Read the model definition and answer for the solid it produces. Units are mm, in the model's axes. A direction names the side the tool comes from. Coordinates: 2 decimals unless noted, no trailing zeros. Order: outer loops, then holes, each group sorted by start corner. A loop starts at its lowest first (then second) coordinate and runs counter-clockwise, first axis right, second up.
```python
from build123d import *

# Parameters (mm, degrees)
SKETCH_1_W        = 120
SKETCH_1_H        = 80
SKETCH_1_W_2      = 28
SKETCH_1_H_2      = 45
BASE_PLATE_DEPTH  = 4
TABS2_START       = -5
TABS2_DEPTH       = 10
TABS2_2_OUTLINE_W = 26
TABS2_2_OUTLINE_H = 4
TABS2_2_DEPTH     = 1.41096
TABS2_START_2     = 5
TABS2_3_OUTLINE_W = 26
TABS2_3_OUTLINE_H = 4
TABS2_3_DEPTH     = 20
TABS2_START_3     = -13
TABS2_4_DEPTH     = 26
TABS2_5_DEPTH     = 26
HOLES_DEPTH       = 77.321687612
HOLES_DEPTH_BACK  = 77.321687612
SKETCH_10_R       = 4.05
SKETCH_12_W       = 8.2
SKETCH_12_H       = 8.2
HOLE2_DEPTH       = 4
FILLET_2_R        = 10
SKETCH_11_R       = 5.1
MOUNT_HOLES_DEPTH = 4


with BuildPart() as part:
    # Base Plate: sheet metal written as solids
    # Sketch 1 → Base Plate (new body)
    with BuildSketch(Plane.XY):
        Rectangle(SKETCH_1_W, SKETCH_1_H)
        Rectangle(SKETCH_1_W_2, SKETCH_1_H_2, mode=Mode.SUBTRACT)
    extrude(amount=-BASE_PLATE_DEPTH)

    # Tabs2: read off the stored shape, not the designer's step
    # Tabs2 outline → Tabs2 (cut)
    with BuildSketch(Plane.XY.offset(TABS2_START)):
        with BuildLine():
            ThreePointArc((-13, 31.6), (-13.5, 32.1), (-14, 31.6))
            Line((-14, 31.6), (-14, 22.5))
            Line((-14, 22.5), (-13, 22.5))
            Line((-13, 22.5), (-13, 31.6))
        make_face()
        with BuildLine():
            Line((-13, -22.5), (-14, -22.5))
            Line((-14, -22.5), (-14, -31.6))
            ThreePointArc((-14, -31.6), (-13.5, -32.1), (-13, -31.6))
            Line((-13, -31.6), (-13, -22.5))
        make_face()
        with BuildLine():
            Line((13, 31.6), (13, 22.5))
            Line((13, 22.5), (14, 22.5))
            Line((14, 22.5), (14, 31.6))
            ThreePointArc((14, 31.6), (13.5, 32.1), (13, 31.6))
        make_face()
        with BuildLine():
            Line((14, -22.5), (13, -22.5))
            Line((13, -22.5), (13, -31.6))
            ThreePointArc((13, -31.6), (13.5, -32.1), (14, -31.6))
            Line((14, -31.6), (14, -22.5))
        make_face()
    extrude(amount=TABS2_DEPTH, mode=Mode.SUBTRACT)

    # Tabs2 2 outline → Tabs2 2 (cut)
    with BuildSketch(Plane.XY.offset(TABS2_START)):
        with Locations((0, 24.5)):
            Rectangle(TABS2_2_OUTLINE_W, TABS2_2_OUTLINE_H)
        with Locations((0, -24.5)):
            Rectangle(TABS2_2_OUTLINE_W, TABS2_2_OUTLINE_H)
    extrude(amount=TABS2_2_DEPTH, mode=Mode.SUBTRACT)

    # Tabs2 4 outline → Tabs2 4 (cut)
    with BuildSketch(Plane.YZ.offset(TABS2_START_3)):
        with BuildLine():
            ThreePointArc((31.5, -4), (27.257359313, -2.937253933), (24.016685226, 0))
            Line((24.016685226, 0), (22.5, 0))
            Line((22.5, 0), (22.5, -3.58904))
            Line((22.5, -3.58904), (26.5, -3.58904))
            Line((26.5, -3.58904), (26.5, -4))
            Line((26.5, -4), (31.5, -4))
        make_face()
        with BuildLine():
            Line((-22.5, -3.58904), (-22.5, 0))
            Line((-22.5, 0), (-24.016685226, 0))
            ThreePointArc((-24.016685226, 0), (-27.257359313, -2.937253933), (-31.5, -4))
            Line((-31.5, -4), (-26.5, -4))
            Line((-26.5, -4), (-26.5, -3.58904))
            Line((-26.5, -3.58904), (-22.5, -3.58904))
        make_face()
    extrude(amount=TABS2_4_DEPTH, mode=Mode.SUBTRACT)



with BuildPart() as body_2:
    # Tabs2 3 outline → Tabs2 3 (new body)
    with BuildSketch(Plane.XY.offset(TABS2_START_2)):
        with Locations((0, 24.5)):
            Rectangle(TABS2_3_OUTLINE_W, TABS2_3_OUTLINE_H)
        with Locations((0, -24.5)):
            Rectangle(TABS2_3_OUTLINE_W, TABS2_3_OUTLINE_H)
    extrude(amount=TABS2_3_DEPTH)


with BuildPart() as part_1:
    add(part.part)

    add(body_2.part)  # Tabs2 5 merges body 2
    # Tabs2 5 outline → Tabs2 5 (add)
    with BuildSketch(Plane.YZ.offset(TABS2_START_3)):
        with BuildLine():
            Line((26.5, 5), (22.5, 5))
            ThreePointArc((22.5, 5), (22.88751392, 2.38751392), (24.016685226, 0))
            Line((24.016685226, 0), (31.5, 0))
            ThreePointArc((31.5, 0), (27.964466094, 1.464466094), (26.5, 5))
        make_face()
        with BuildLine():
            Line((-31.5, 0), (-24.016685226, 0))
            ThreePointArc((-24.016685226, 0), (-22.88751392, 2.38751392), (-22.5, 5))
            Line((-22.5, 5), (-26.5, 5))
            ThreePointArc((-26.5, 5), (-27.964466094, 1.464466094), (-31.5, 0))
        make_face()
    extrude(amount=TABS2_5_DEPTH)

    # Эскиз10 → Holes (cut, two sides: drawn at the far end of the back side and taken through both)
    with BuildSketch(Plane(origin=(0, 0, 0), x_dir=(1, 0, 0), z_dir=(0, 1, 0)).offset(-HOLES_DEPTH_BACK)):
        with Locations(Location((0, -17, 0), (0, 0, 90))):
            Circle(SKETCH_10_R)
    extrude(amount=HOLES_DEPTH + HOLES_DEPTH_BACK, mode=Mode.SUBTRACT)

    # Эскиз12 → Hole2 (cut)
    with BuildSketch(Plane(origin=(0, 26.5, 0), x_dir=(1, 0, 0), z_dir=(0, 1, 0))):
        with Locations((0, -17)):
            Rectangle(SKETCH_12_W, SKETCH_12_H)
    extrude(amount=-HOLE2_DEPTH, mode=Mode.SUBTRACT)

    # Fillet 2
    fillet_2_edges = [part_1.edges().sort_by_distance(p)[0] for p in [
        (13, -24.5, 25),
        (-13, -24.5, 25),
        (-60, 40, -2),
        (60, 40, -2),
        (60, -40, -2),
        (-60, -40, -2),
        (-13, 24.5, 25),
        (13, 24.5, 25),
    ]]
    fillet(fillet_2_edges, radius=FILLET_2_R)

    # Эскиз11 → Mount Holes (cut)
    with BuildSketch(Plane.XY):
        with Locations((-45, 25)):
            Circle(SKETCH_11_R)
        with Locations((45, 25)):
            Circle(SKETCH_11_R)
        with Locations((-45, -25)):
            Circle(SKETCH_11_R)
        with Locations((45, -25)):
            Circle(SKETCH_11_R)
    extrude(amount=-MOUNT_HOLES_DEPTH, mode=Mode.SUBTRACT)


solid = part_1.part
```
1) Which of the six approach directions +Z, -Z, +X, -X, +Y, -Y give full straight-line access (tool end or side, diameter ignored) to faces 1 (the flat face through (-14.2, 0.6, -4)), 2 (the flat face through (-0.2, -22.5, 12.6)), 3 (the flat face through (-14, 0, -2))?
A:
face 1: -Z, +X, -X, +Y, -Y
face 2: +Z, -Z, +X, -X
face 3: +Z, -Z
2) Determine the mould class of faces 4 (the cylindrical face through (56.99, 37.15, -2.03)), 5 (the flat face through (4.1, 25, 17)), 6 (the flat face through (14, 0, -2)), 7 (the flat face through (-14.2, 0.6, 0)) for opening direction X: pulls with the +X half, pulls with the -X half, needs draft (parallel to the pull), parting line crosses it, or undercut.
A:
face 4: pulls with the +X half
face 5: undercut
face 6: undercut
face 7: needs draft
3) A cutting plane is placed at D-D, the plane x = 45. Determine the outline of the cut face in (y, z), and give its area (3 significant figures).
A:
outline: (-40, -4) - (-30.1, -4) - (-30.1, 0) - (-40, 0) - close; (-19.9, -4) - (19.9, -4) - (19.9, 0) - (-19.9, 0) - close; (30.1, -4) - (40, -4) - (40, 0) - (30.1, 0) - close
area: 238 mm2
4) Flat-ended cylindrical pins translate along their axes: pin 1 Ø3 at (x, y) = (-39.5, -12) entering from +Z; pin 2 Ø5 at (y, z) = (12.5, 4.5) entering from -X; pin 3 Ø4.5 at (y, z) = (-26, 6) entering from +X; pin 4 Ø9.5 at (x, z) = (0, 17) entering from +Y. Find the tip coordinate at first contact, or state that the pin passes through.
A:
pin 1: stops at z = 0
pin 2: passes through
pin 3: stops at x = 13
pin 4: stops at y = 26.5
5) A cutting plane is placed at B-B, the plane y = 8. Determine the outline of the cut face in (x, z), and give its area (3 significant figures).
A:
outline: (-60, -4) - (-14, -4) - (-14, 0) - (-60, 0) - close; (14, -4) - (60, -4) - (60, 0) - (14, 0) - close
area: 368 mm2
6) Straight lines are drawn through the part: line 1 (Y direction, x = -45, z = -1.1); line 2 (X direction, y = 9.5, z = -2.5); line 3 (Y direction, x = -6, z = 18.5). For each, find the intervals that lie inside material, in ascending order.
A:
line 1: y = -40 to -30.1, -19.9 to 19.9, 30.1 to 40
line 2: x = -60 to -14, 14 to 60
line 3: y = -26.5 to -22.5, 22.5 to 26.5
7) A cutting plane is placed at C-C, the plane z = 3.25. Determine the outline of the cut face in (x, y), and give its area (3 significant figures).
A:
outline: (-13, -26.82) - (13, -26.82) - (13, -22.67) - (-13, -22.67) - close; (-13, 22.67) - (13, 22.67) - (13, 26.82) - (-13, 26.82) - close
area: 216 mm2
8) A cutting plane is placed at A-A, the plane x = 0. Determine the outline of the cut face in (y, z).
A:
outline: (-40, -4) - (-31.5, -4) arc R9 ccw to (-22.5, 5) - (-22.5, 12.95) - (-26.5, 12.95) - (-26.5, 5) arc R5 cw to (-31.5, 0) - (-40, 0) - close; (-26.5, 21.05) - (-22.5, 21.05) - (-22.5, 25) - (-26.5, 25) - close; (22.5, 5) arc R9 ccw to (31.5, -4) - (40, -4) - (40, 0) - (31.5, 0) arc R5 cw to (26.5, 5) - (26.5, 12.9) - (22.5, 12.9) - close; (22.5, 21.1) - (26.5, 21.1) - (26.5, 25) - (22.5, 25) - close
